from build123d import *

# Parameters (mm, degrees)
F0_R     = 5.08
F1_DEPTH = 17.78
F2_R     = 5.08
F2_R_2   = 3.683
F3_DEPTH = 6.35
F4_R     = 5.08
F4_R_2   = 3.81
F5_DEPTH = 5.08
F6_R     = 3.81
F7_DEPTH = 5.08
F8_R     = 3.683
F9_DEPTH = 1.27


# Not quite as in the source:
# - a fillet or chamfer that OpenCascade refuses, or shapes differently, is made with other operations: its cross-section is extruded or revolved along the edge and cut away or added


with BuildPart() as f1:
    # F0 (on Right) → F1 (new body)
    with BuildSketch(Plane.YZ):
        Circle(F0_R)
    extrude(amount=F1_DEPTH)

    # F2 (on face) → F3 (cut)
    with BuildSketch(Plane(origin=(0, 0, 0), x_dir=(0, -1, 0), z_dir=(-1, 0, 0))):
        Circle(F2_R)
        Circle(F2_R_2, mode=Mode.SUBTRACT)
    extrude(amount=-F3_DEPTH, mode=Mode.SUBTRACT)

    # F4 (on face) → F5 (cut)
    with BuildSketch(Plane(origin=(6.35, 0, 0), x_dir=(0, -1, 0), z_dir=(-1, 0, 0))):
        Circle(F4_R)
        Circle(F4_R_2, mode=Mode.SUBTRACT)
    extrude(amount=-F5_DEPTH, mode=Mode.SUBTRACT)

    # F6 (on face) → F7 (cut)
    with BuildSketch(Plane.YZ.offset(17.78)):
        Circle(F6_R)
    extrude(amount=-F7_DEPTH, mode=Mode.SUBTRACT)

    # F8 (on face) → F9 (cut)
    with BuildSketch(Plane(origin=(0, 0, 0), x_dir=(0, -1, 0), z_dir=(-1, 0, 0))):
        Circle(F8_R)
    extrude(amount=-F9_DEPTH, mode=Mode.SUBTRACT)

    # F10: fillet of radius 2.54 on 1 edges, made by hand

    # F10_s1 → F10_t2 (revolve, cut)
    with BuildSketch(Plane.XY):
        with BuildLine():
            ThreePointArc((15.5802954744, 5.08), (16.8502954744, 4.7397045256), (17.78, 3.81))
            Line((17.78, 3.81), (17.78, 5.08))
            Line((17.78, 5.08), (15.5802954744, 5.08))
        make_face()
    revolve(axis=Axis((17.78, 0, 0), (1, 0, 0)), mode=Mode.SUBTRACT)


solid = f1.part
Geometry: final body of the model. Coordinates: model frame, mm. A direction names the side the tool comes from. Coordinates: 2 decimals unless noted, no trailing zeros. Loops run counter-clockwise (first coordinate to the right, second up) from the corner with the lowest first, then second, coordinate; pieces in that order, holes last. Notation, with made-up numbers: (89, 37) - (130, 37) arc R25 cw to (130, 56) - close; hole circle Ø1 at (16, 41). An arc over 180 degrees is marked (long way). Put each result on its own line as item: value. Start each with the question number.
Q1. Set-up query: faces 4 (the flat face through (1.27, 0, 0)), 5 (the flat face through (12.7, 0, 0)), 6 (the cylindrical face through (3.774, -1.699, -3.267)). Return all of +Z, -Z, +X, -X, +Y, -Y with unobstructed straight access to the full face (end or side cutting, diameter ignored); none if empty.
Q2. Cut plane C-C, the plane x = 10.5. Return loops of the section in (y, z), and give its area (3 significant figures).
Q3. Cut plane A-A, the plane x = 14. Return loops of the section in (y, z).
Q4. Pin query (flat end, axial travel): pin 1 Ø2 at (x, z) = (15.5, 2.5) entering from +Y; pin 2 Ø1.5 at (y, z) = (3.5, 3) entering from -X; pin 3 Ø1 at (x, y) = (9, 0.5) entering from +Z; pin 4 Ø4 at (y, z) = (1, 3.5) entering from +X. Return the tip coordinate at first contact, or that it passes through.
Q5. Pull-direction query (Y, two-part tool) for faces 1 (the cylindrical face through (15.28, -0.83, -3.72)), 2 (the flat face through (11.43, -1, 4)), 3 (the cylindrical face through (8.85, 0.83, -3.72)); classes: released by +Y, released by -Y, zero draft, split by the parting line, or undercut.
Q6. Cut plane B-B, the plane x = 5. Return loops of the section in (y, z).
Q7. Line query: line 1 (Z direction, x = 15.7, y = 0); line 2 (X direction, y = -0.75, z = -1); line 3 (Z direction, x = 12.75, y = -1.75). Output: solid intervals per line, ascending.
Filled sheet:
1. face 4: +Z, -Z, -X, +Y, -Y
1. face 5: +X
1. face 6: -X
2. outline: circle Ø7.62 at (0, 0)
2. area: 45.6 mm²
3. outline: circle Ø10.16 at (0, 0); hole circle Ø7.62 at (0, 0)
4. pin 1: y = 4.85
4. pin 2: x = 11.43
4. pin 3: z = 3.81
4. pin 4: x = 17.78
5. face 1: undercut
5. face 2: zero draft
5. face 3: split by the parting line
6. outline: circle Ø7.37 at (0, 0)
7. line 1: -5.08 to -3.81, 3.81 to 5.08
7. line 2: 1.27 to 12.7
7. line 3: -4.77 to -3.38, 3.38 to 4.77
